Source: three-view drawing plus pictorial views. Frame: mm from the lowest corner of the part. Give positions to 0.01 mm unless a question says otherwise; leave off trailing zeros. Loops run counter-clockwise (first coordinate to the right, second up) from the corner with the lowest first, then second, coordinate; pieces in that order, holes last. Notation, with made-up numbers: (46, -28.75) - (63, -28.75) arc R25 ccw to (63, -13.75) - close; hole circle Ø9 at (33, -33.5). An arc over 180 degrees is marked (long way). Answer in a Markdown table with one row per item.
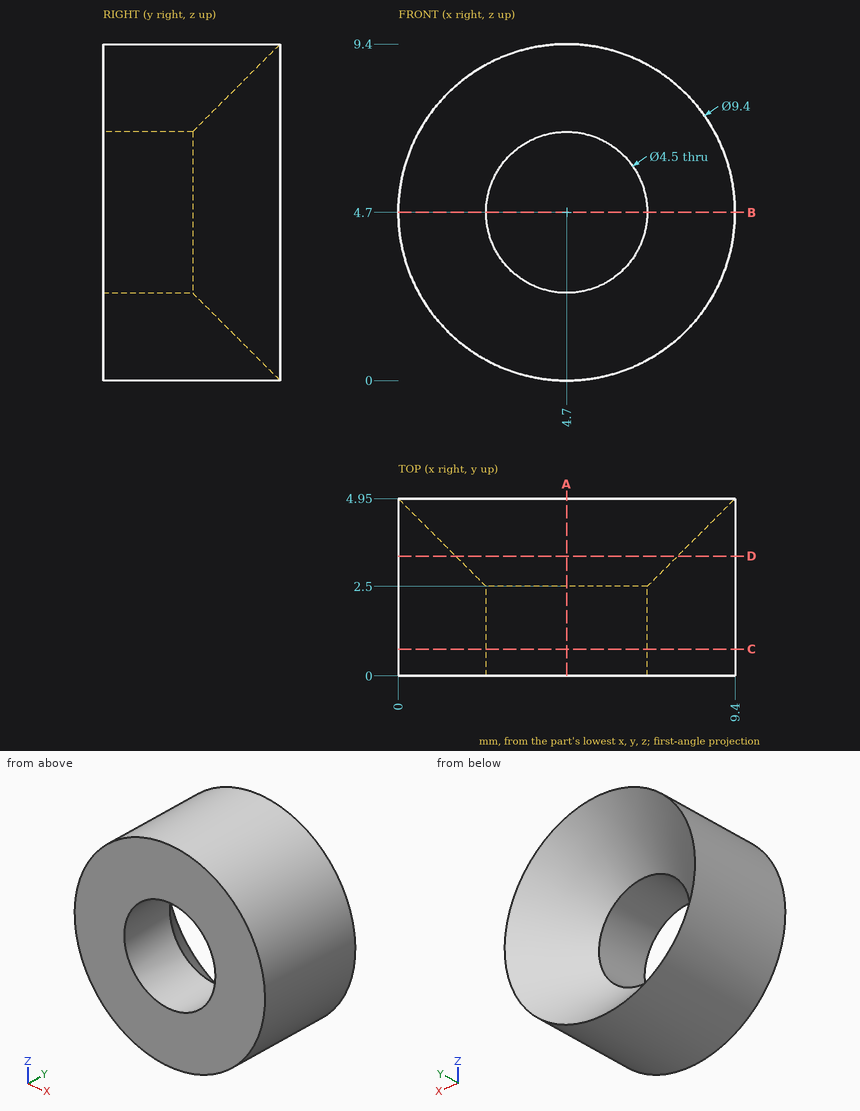
Q1. Material intervals for line 1 along X through (y, z) = (1.6, 4.7); line 2 along X through (y, z) = (4.3, 2.5); line 3 along Z through (x, y) = (3.5, 2.35), sorted ascending.
Check values:
| item | result |
|---|---|
| line 1 | 0 to 2.45, 6.95 to 9.4 |
| line 2 | 0.55 to 1.3, 8.1 to 8.85 |
| line 3 | 0.16 to 2.8, 6.6 to 9.24 |
Q2. Cut plane D-D (y = 3.35). Output: boundary loops of the cut face in (x, z).
Check values:
| item | result |
|---|---|
| outline | circle Ø9.4 at (4.7, 4.7); hole circle Ø6.2 at (4.7, 4.7) |
Q3. First-contact query: pin 1 (1 mm diameter, centred on y = 1.5, z = 4, fed in from +X); pin 2 (3.5 mm diameter, centred on x = 4.7, z = 4.7, fed in from +Y); pin 3 (1.5 mm diameter, centred on y = 2, z = 2.5, fed in from -X). Flat tips, straight axial feed; report the tip coordinate or a pass-through.
Check values:
| item | result |
|---|---|
| pin 1 | x = 9.4 |
| pin 2 | through |
| pin 3 | x = 0.23 |
Q4. Cut plane B-B (z = 4.7). Output: boundary loops of the cut face in (x, y).
Check values:
| item | result |
|---|---|
| outline | (0, 0) - (2.45, 0) - (2.45, 2.5) - (0, 4.95) - close; (6.95, 0) - (9.4, 0) - (9.4, 4.95) - (6.95, 2.5) - close |
Q5. Cut plane C-C (y = 0.75). Output: boundary loops of the cut face in (x, z).
Check values:
| item | result |
|---|---|
| outline | circle Ø9.4 at (4.7, 4.7); hole circle Ø4.5 at (4.7, 4.7) |
Q6. Cut plane A-A (x = 4.7). Output: boundary loops of the cut face in (y, z).
Check values:
| item | result |
|---|---|
| outline | (0, 0) - (4.95, 0) - (2.5, 2.45) - (0, 2.45) - close; (0, 6.95) - (2.5, 6.95) - (4.95, 9.4) - (0, 9.4) - close |
